Verification items for the finished model (mm, model axes). Give positions to 0.01 mm unless a question says otherwise; leave off trailing zeros. Write each loop counter-clockwise with the first axis right and the second up, starting at its lowest first coordinate (ties: lowest second). Pieces come first, ordered by that corner, then holes. Notation, with made-up numbers: (58, 37.25) -> (74, 37.25) arc R14 cw to (74, 52.25) -> close; hole circle Ø4 at (10.25, -21). An arc over 180 degrees is marked (long way). Write item = value, one per line.
from build123d import *

# Parameters (mm, degrees)
ESQUISSE1_R             = 5
ESQUISSE1_R_2           = 2
BOSS_EXTRU_1_DEPTH      = 3
ESQUISSE3_W             = 3
ESQUISSE3_H             = 10
ESQUISSE3_W_2           = 10
ESQUISSE3_H_2           = 3
ENL_V_MAT_EXTRU_1_DEPTH = 165.022412006


with BuildPart() as part:
    # Esquisse1 → Boss.-Extru.1 (new body)
    with BuildSketch(Plane.XY):
        with BuildLine():
            Line((78.109352882, -135), (-41.890647118, -135))
            Line((-41.890647118, -135), (-41.890647118, 5))
            Line((-41.890647118, 5), (-26.890647118, 5))
            Line((-26.890647118, 5), (-26.890647118, 41.795417818))
            Line((-26.890647118, 41.795417818), (-56.890647118, 41.795417818))
            add(Edge.make_bspline(
                [(-56.890647118, 41.795417818), (-56.746915478, 58.294848354), (-44.215904994, 62.728898217)],
                knots=[0, 0, 0, 1, 1, 1], degree=2))
            add(Edge.make_bspline(
                [(-44.215904994, 62.728898217), (-30.528185851, 67.934087187), (18.109352882, 68.550704045)],
                knots=[0, 0, 0, 1, 1, 1], degree=2))
            add(Edge.make_bspline(
                [(80.434610758, 62.728898217), (66.746891614, 67.934087187), (18.109352882, 68.550704045)],
                knots=[0, 0, 0, 1, 1, 1], degree=2))
            add(Edge.make_bspline(
                [(93.109352882, 41.795417818), (92.965621241, 58.294848354), (80.434610758, 62.728898217)],
                knots=[0, 0, 0, 1, 1, 1], degree=2))
            Line((93.109352882, 41.795417818), (63.109352882, 41.795417818))
            Line((63.109352882, 41.795417818), (63.109352882, 5))
            Line((63.109352882, 5), (78.109352882, 5))
            Line((78.109352882, 5), (78.109352882, -135))
        make_face()
        with Locations((18.109352882, 10.811644987)):
            Circle(ESQUISSE1_R, mode=Mode.SUBTRACT)
        with Locations((18.109352882, 53.550704045)):
            Circle(ESQUISSE1_R_2, mode=Mode.SUBTRACT)
        with Locations((-8.390647118, 53.550704045)):
            Circle(ESQUISSE1_R_2, mode=Mode.SUBTRACT)
        with Locations((-34.390647118, 53.550704045)):
            Circle(ESQUISSE1_R_2, mode=Mode.SUBTRACT)
        with Locations(Location((70.609352882, 53.550704045, 0), (0, 0, 180))):
            Circle(ESQUISSE1_R_2, mode=Mode.SUBTRACT)
        with Locations(Location((44.609352882, 53.550704045, 0), (0, 0, 180))):
            Circle(ESQUISSE1_R_2, mode=Mode.SUBTRACT)
        with Locations((18.109352882, 61.055482272)):
            Circle(ESQUISSE1_R_2, mode=Mode.SUBTRACT)
        with Locations((-21.390647118, 53.550704045)):
            Circle(ESQUISSE1_R_2, mode=Mode.SUBTRACT)
        with Locations(Location((57.609352882, 53.550704045, 0), (0, 0, 180))):
            Circle(ESQUISSE1_R_2, mode=Mode.SUBTRACT)
    extrude(amount=BOSS_EXTRU_1_DEPTH)

    # Esquisse3 → Enlèv. mat.-Extru.1 (cut, through all)
    with BuildSketch(Plane.XY.offset(3)):
        with Locations((-22.390647118, -115)):
            Rectangle(ESQUISSE3_W, ESQUISSE3_H)
        with Locations((-22.390647118, -90)):
            Rectangle(ESQUISSE3_W, ESQUISSE3_H)
        with Locations((-22.390647118, -65)):
            Rectangle(ESQUISSE3_W, ESQUISSE3_H)
        with Locations((-22.390647118, -40)):
            Rectangle(ESQUISSE3_W, ESQUISSE3_H)
        with Locations((-22.390647118, -15)):
            Rectangle(ESQUISSE3_W, ESQUISSE3_H)
        with Locations((-22.390647118, 10)):
            Rectangle(ESQUISSE3_W, ESQUISSE3_H)
        with Locations((-22.390647118, 35)):
            Rectangle(ESQUISSE3_W, ESQUISSE3_H)
        with Locations((58.609352882, -15)):
            Rectangle(ESQUISSE3_W, ESQUISSE3_H)
        with Locations((58.609352882, 10)):
            Rectangle(ESQUISSE3_W, ESQUISSE3_H)
        with Locations((58.609352882, 35)):
            Rectangle(ESQUISSE3_W, ESQUISSE3_H)
        with Locations((58.609352882, -65)):
            Rectangle(ESQUISSE3_W, ESQUISSE3_H)
        with Locations((58.609352882, -40)):
            Rectangle(ESQUISSE3_W, ESQUISSE3_H)
        with Locations((58.609352882, -90)):
            Rectangle(ESQUISSE3_W, ESQUISSE3_H)
        with Locations((58.609352882, -115)):
            Rectangle(ESQUISSE3_W, ESQUISSE3_H)
        with Locations((-6.890647118, 42.5)):
            Rectangle(ESQUISSE3_W_2, ESQUISSE3_H_2)
        with Locations((18.109352882, 42.5)):
            Rectangle(ESQUISSE3_W_2, ESQUISSE3_H_2)
        with Locations((43.109352882, 42.5)):
            Rectangle(ESQUISSE3_W_2, ESQUISSE3_H_2)
    extrude(amount=-ENL_V_MAT_EXTRU_1_DEPTH, mode=Mode.SUBTRACT)


solid = part.part
Item 1: Sectioned sample at C-C on z = 0.65. Give the number of separate pieces and of enclosed holes in the cut face, then the cut area to 3 significant figures.
Response values:
separate_pieces = 1
enclosed_holes = 26
area = 23,000 mm^2
Item 2: Sectioned sample at D-D on y = 27.5. Record the cut outline in (x, z).
Response values:
outline = (-26.89, 0) -> (63.11, 0) -> (63.11, 3) -> (-26.89, 3) -> close
Item 3: Mould release check, pull along X, two halves, no side actions. Record for faces 1 (the cylindrical face through (46.083, 52.199, 1.479)), 2 (the flat face through (19, -32, 0)): +X half, -X half, draft (parallel to the pull), parting line (faces both ways), or undercut.
Response values:
face_1 = undercut
face_2 = draft
Item 4: Go/stop test with flat-tipped pins: P1, Ø0.9, axis at x = -32, z = 1, coming from the +Y side; P2, Ø1, axis at x = 13, z = 1, coming from the +Y side; P3, Ø1.5, axis at y = -73, z = 1, coming from the +X side. Record where each tip stops, or that it passes through.
Response values:
P1 = 65.64
P2 = 68.48
P3 = 78.11
Item 5: Material ranges on line 1 (X direction, y = -65, z = 1.5); line 2 (X direction, y = 38, z = 0.3); line 3 (Y direction, x = 18.5, z = 0.6), recorded low to high.
Response values:
line_1 = -41.89 to -23.89, -20.89 to 57.11, 60.11 to 78.11
line_2 = -26.89 to -23.89, -20.89 to 57.11, 60.11 to 63.11
line_3 = -135 to 5.83, 15.8 to 41, 44 to 51.59, 55.51 to 59.09, 63.02 to 68.55
Item 6: Sectioned sample at A-A on y = -12.5. Record the cut outline in (x, z), then the cut area to 3 significant figures.
Response values:
outline = (-41.89, 0) -> (-23.89, 0) -> (-23.89, 3) -> (-41.89, 3) -> close; (-20.89, 0) -> (57.11, 0) -> (57.11, 3) -> (-20.89, 3) -> close; (60.11, 0) -> (78.11, 0) -> (78.11, 3) -> (60.11, 3) -> close
area = 342 mm^2
Item 7: Sectioned sample at B-B on y = -81. Record the cut outline in (x, z), then the cut area to 3 significant figures.
Response values:
outline = (-41.89, 0) -> (78.11, 0) -> (78.11, 3) -> (-41.89, 3) -> close
area = 360 mm^2
